Build history of the part. All positions in model axes, mm. A direction names the side the tool comes from. Round coordinates to 2 decimals unless told otherwise and drop trailing zeros. Write each loop counter-clockwise with the first axis right and the second up, starting at its lowest first coordinate (ties: lowest second). Pieces come first, ordered by that corner, then holes.
from build123d import *

# Parameters (mm, degrees)
SKETCH_1_W          = 30
SKETCH_1_H          = 6
EXTRUDE_1_DEPTH     = 24
SKETCH_2_W          = 16
SKETCH_2_H          = 6
CUT_EXTRUDE_1_DEPTH = 45.777226354
SKETCH_3_W          = 4
SKETCH_3_H          = 4
EXTRUDE_2_DEPTH     = 30
SKETCH_4_W          = 26
SKETCH_4_H          = 4
EXTRUDE_3_DEPTH     = 10
SKETCH_5_W          = 4
SKETCH_5_H          = 10
CUT_EXTRUDE_3_DEPTH = 47.957427527
SKETCH_6_W          = 4
SKETCH_6_H          = 10
CUT_EXTRUDE_5_DEPTH = 47.957427527
SKETCH_7_R          = 4
EXTRUDE_5_DEPTH     = 30
SKETCH_8_R          = 4
CUT_EXTRUDE_6_DEPTH = 4
SKETCH_9_R          = 4
CUT_EXTRUDE_7_DEPTH = 44.324358045
SKETCH_10_W         = 3.23
SKETCH_10_H         = 3.54
EXTRUDE_6_DEPTH     = 30
SKETCH_11_W         = 3.23
SKETCH_11_H         = 3.54
CUT_EXTRUDE_8_DEPTH = 45.777226354
EXTRUDE_7_DEPTH     = 30


with BuildPart() as part:
    # 草图1 → 凸台-拉伸1 (new body)
    with BuildSketch(Plane.XY):
        Polygon((15, 23), (-15, -17), (15, -17), align=None)
        with Locations((0, -20)):
            Rectangle(SKETCH_1_W, SKETCH_1_H)
    extrude(amount=EXTRUDE_1_DEPTH)

    # 草图2 → 切除-拉伸1 (cut, through all)
    with BuildSketch(Plane.ZY.offset(15)):
        with Locations((12, -20)):
            Rectangle(SKETCH_2_W, SKETCH_2_H)
    extrude(amount=-CUT_EXTRUDE_1_DEPTH, mode=Mode.SUBTRACT)

    # 草图3 → 凸台-拉伸2 (add)
    with BuildSketch(Plane.ZY.offset(15)):
        with Locations((2, -25)):
            Rectangle(SKETCH_3_W, SKETCH_3_H)
        with Locations((22, -25)):
            Rectangle(SKETCH_3_W, SKETCH_3_H)
    extrude(amount=-EXTRUDE_2_DEPTH)

    # 草图4 → 凸台-拉伸3 (add)
    with BuildSketch(Plane.XZ.offset(17)):
        with Locations((-2, 12)):
            Rectangle(SKETCH_4_W, SKETCH_4_H)
    extrude(amount=EXTRUDE_3_DEPTH)

    # 草图5 → 切除-拉伸3 (cut, through all)
    with BuildSketch(Plane(origin=(15, 0, 0), x_dir=(0, 0, -1), z_dir=(1, 0, 0))):
        with Locations((-2, -22)):
            Rectangle(SKETCH_5_W, SKETCH_5_H)
        with Locations((-22, -22)):
            Rectangle(SKETCH_5_W, SKETCH_5_H)
    extrude(amount=-CUT_EXTRUDE_3_DEPTH, mode=Mode.SUBTRACT)

    # 草图6 → 切除-拉伸5 (cut, through all)
    with BuildSketch(Plane.ZY.offset(15)):
        with Locations((12, -22)):
            Rectangle(SKETCH_6_W, SKETCH_6_H)
    extrude(amount=-CUT_EXTRUDE_5_DEPTH, mode=Mode.SUBTRACT)

    # 草图10 → 凸台-拉伸6 (add)
    with BuildSketch(Plane(origin=(15, 0, 0), x_dir=(0, 0, -1), z_dir=(1, 0, 0))):
        with Locations((-12, -18.77)):
            Rectangle(SKETCH_10_W, SKETCH_10_H)
    extrude(amount=-EXTRUDE_6_DEPTH)

    # 草图11 → 切除-拉伸8 (cut, through all)
    with BuildSketch(Plane(origin=(15, 0, 0), x_dir=(0, 0, -1), z_dir=(1, 0, 0))):
        with Locations((-12, -18.77)):
            Rectangle(SKETCH_11_W, SKETCH_11_H)
    extrude(amount=-CUT_EXTRUDE_8_DEPTH, mode=Mode.SUBTRACT)

    # 草图12 → 凸台-拉伸7 (add)
    with BuildSketch(Plane(origin=(15, 0, 0), x_dir=(0, 0, -1), z_dir=(1, 0, 0))):
        Polygon((-13.767766953, -20.23), (-12, -21.997766953), (-10.232233047, -20.23), align=None)
        with BuildLine():
            Line((-10.232233047, -20.23), (-12, -21.997766953))
            Line((-12, -21.997766953), (-13.767766953, -20.23))
            ThreePointArc((-13.767766953, -20.23), (-12.956708581, -24.307465784), (-9.5, -21.997766953))
            ThreePointArc((-9.5, -21.997766953), (-9.690301169, -21.041058372), (-10.232233047, -20.23))
        make_face()
        with BuildLine():
            ThreePointArc((-13.767766953, -20.23), (-12, -19.497766953), (-10.232233047, -20.23))
            Line((-10.232233047, -20.23), (-10.232233047, -17))
            Line((-10.232233047, -17), (-13.767766953, -17))
            Line((-13.767766953, -17), (-13.767766953, -20.23))
        make_face()
        with BuildLine():
            Line((-13.767766953, -20.23), (-10.232233047, -20.23))
            ThreePointArc((-10.232233047, -20.23), (-12, -19.497766953), (-13.767766953, -20.23))
        make_face()
    extrude(amount=-EXTRUDE_7_DEPTH)


with BuildPart() as body_2:
    # 草图7 → 凸台-拉伸5 (new body)
    with BuildSketch(Plane(origin=(15, 0, 0), x_dir=(0, 0, -1), z_dir=(1, 0, 0))):
        with Locations((-12, -21)):
            Circle(SKETCH_7_R)
    extrude(amount=-EXTRUDE_5_DEPTH)

    # 草图8 → 切除-拉伸6 (cut)
    with BuildSketch(Plane(origin=(15, 0, 0), x_dir=(0, 0, -1), z_dir=(1, 0, 0))):
        with Locations((-12, -21)):
            Circle(SKETCH_8_R)
    extrude(amount=-CUT_EXTRUDE_6_DEPTH, mode=Mode.SUBTRACT)

    # 草图9 → 切除-拉伸7 (cut, through all)
    with BuildSketch(Plane(origin=(11, 0, 0), x_dir=(0, 0, -1), z_dir=(1, 0, 0))):
        with Locations((-12, -21)):
            Circle(SKETCH_9_R)
    extrude(amount=-CUT_EXTRUDE_7_DEPTH, mode=Mode.SUBTRACT)


solid = part.part
1) Which spindle directions (+Z, -Z, +X, -X, +Y, -Y) get a long thin tool onto all of the face, cutting with end or side? Do faces 1 (the flat face through (6, -6, 24)), 2 (the flat face through (0, -19, 10.232)). Say none if no direction does.
Results:
face 1: +Z, +X, -X, +Y, -Y
face 2: -Z, +X, -X
2) Wall check: L1, parallel to Y at x = -10.5, z = 10; L2, parallel to Y at x = 7.75, z = 7; L3, parallel to X at y = 14, z = 16. Give the ranges that are in metal, low to high.
Results:
L1: y = -23.5 to -20.5, -17 to -11
L2: y = -17 to 13.33
L3: x = 8.25 to 15
3) Slice it at A-A (x = 7.5). Write the cut outline in (y, z).
Results:
outline: (-20.23, 10.23) - (-17, 10.23) - (-17, 0) - (13, 0) - (13, 24) - (-17, 24) - (-17, 13.77) - (-20.23, 13.77) arc R2.5 ccw (long way) to start
4) Pin check, flat tips, straight feed: pin 1 Ø3 at (x, z) = (-4, 3.5) entering from -Y; pin 2 Ø3 at (x, z) = (-11.5, 21) entering from +Y; pin 3 Ø12 at (x, z) = (3, 18.5) entering from -Y. Stop position of each tip, or through.
Results:
pin 1: stops at y = -17
pin 2: stops at y = -10.33
pin 3: stops at y = -24.45
5) Slice it at B-B (y = -11). Write the cut outline in (x, z).
Results:
outline: (-10.5, 0) - (15, 0) - (15, 24) - (-10.5, 24) - close
6) Slice it at D-D (z = 12). Write the cut outline in (x, y), plus the area to 3 significant figures.
Results:
outline: (-15, -24.5) - (15, -24.5) - (15, 23) - (-15, -17) - close
area: 825 mm2
7) Mould opens along Y. For faces 3 (the flat face through (0, 3, 12)), 4 (the flat face through (-15, -21, 12)), 5 (the flat face through (0, -19, 13.768)) say: released by +Y, released by -Y, zero draft, split by the parting line, or undercut.
Results:
face 3: released by +Y
face 4: zero draft
face 5: undercut
8) Slice it at C-C (x = 12). Write the cut outline in (y, z).
Results:
outline: (-20.23, 10.23) - (-17, 10.23) - (-17, 0) - (19, 0) - (19, 24) - (-17, 24) - (-17, 13.77) - (-20.23, 13.77) arc R2.5 ccw (long way) to start
